```python
from build123d import *

# Parameters (mm, degrees)
BOSS_EXTRUDE1_DEPTH   = 1
SKETCH4_R             = 2
BOSS_EXTRUDE3_DEPTH   = 0.5
SKETCH2_R             = 1
BOSS_EXTRUDE2_DEPTH   = 0.5
CHAMFER1_SIZE         = 0.254
SKETCH5_W             = 0.790640215
SKETCH5_H             = 0.2205187
BOSS_EXTRUDE4_DEPTH   = 1.644
BOSS_EXTRUDE4_2_DEPTH = 1.644
SKETCH7_W             = 0.790640215
SKETCH7_H             = 0.233563057
BOSS_EXTRUDE5_DEPTH   = 0.6
BOSS_EXTRUDE5_2_DEPTH = 0.6
LOFT1_START           = 1.157491545
LOFT1_DEPTH           = 0.790640215
LOFT2_START           = -2.978578696
LOFT2_DEPTH           = 0.790640215
FILLET1_R             = 0.508


# Read off the part's stored shape, not the designer's step: Loft1, Loft2, Mirror1
with BuildPart() as part:
    # Sketch1 → Boss-Extrude1 (new body)
    with BuildSketch(Plane(origin=(0, 0, 0), x_dir=(1, 0, 0), z_dir=(0, 1, 0))):
        Polygon((-3.115223468, 1.972186251), (-2.070005732, 3.017403987), (1.039558796, 3.017403987), (2.084776532, 1.972186251), (2.084776532, -1.137378277), (1.039558796, -2.182596013), (-2.070005732, -2.182596013), (-3.115223468, -1.137378277), align=None)
    extrude(amount=BOSS_EXTRUDE1_DEPTH)

    # Sketch4 → Boss-Extrude3 (add)
    with BuildSketch(Plane(origin=(0, 1, 0), x_dir=(1, 0, 0), z_dir=(0, 1, 0))):
        with Locations(Location((-0.515223468, 0.417403987, 0), (0, 0, 270))):
            Circle(SKETCH4_R)
    extrude(amount=BOSS_EXTRUDE3_DEPTH)

    # Sketch2 → Boss-Extrude2 (add)
    with BuildSketch(Plane(origin=(0, 1.5, 0), x_dir=(1, 0, 0), z_dir=(0, 1, 0))):
        with Locations(Location((-0.515223468, 0.417403987, 0), (0, 0, 270))):
            Circle(SKETCH2_R)
    extrude(amount=BOSS_EXTRUDE2_DEPTH)

    # Chamfer1
    chamfer1_edges = [part.edges().sort_by_distance(p)[0] for p in [
        (-0.515223468, 1.5, -2.417403987),
    ]]
    chamfer(chamfer1_edges, length=CHAMFER1_SIZE)



with BuildPart() as body_2:
    # Sketch5 → Boss-Extrude4 (new body)
    with BuildSketch(Plane.XY.offset(2.182596013)):
        with Locations((-2.583258589, 0.233563057)):
            Rectangle(SKETCH5_W, SKETCH5_H)
    extrude(amount=-BOSS_EXTRUDE4_DEPTH)



with BuildPart() as body_3:
    # Sketch5 → Boss-Extrude4 2 (new body)
    with BuildSketch(Plane.XY.offset(2.182596013)):
        with Locations((1.552811652, 0.233563057)):
            Rectangle(SKETCH5_W, SKETCH5_H)
    extrude(amount=-BOSS_EXTRUDE4_2_DEPTH)


with BuildPart() as body_4:
    # Sketch7 → Boss-Extrude5 (new body)
    with BuildSketch(Plane.XY.offset(2.436596013)):
        with Locations((-2.583258589, 0.116781529)):
            Rectangle(SKETCH7_W, SKETCH7_H)
    extrude(amount=BOSS_EXTRUDE5_DEPTH)


with BuildPart() as body_5:
    # Sketch7 → Boss-Extrude5 2 (new body)
    with BuildSketch(Plane.XY.offset(2.436596013)):
        with Locations((1.552811652, 0.116781529)):
            Rectangle(SKETCH7_W, SKETCH7_H)
    extrude(amount=BOSS_EXTRUDE5_2_DEPTH)


with BuildPart() as part_1:
    add(part.part)

    add(body_3.part)  # Loft1 merges body 3

    add(body_5.part)  # Loft1 merges body 5
    # Loft1 outline → Loft1 (add)
    with BuildSketch(Plane.YZ.offset(LOFT1_START)):
        Polygon((0.233563057, 2.436596013), (0, 2.436596013), (0.123303707, 2.182596013), (0.343822407, 2.182596013), align=None)
    extrude(amount=LOFT1_DEPTH)


with BuildPart() as body_2_1:
    add(body_2.part)

    add(body_4.part)  # Loft2 merges body 4

    add(part_1.part)  # Loft2 merges part
    # Loft2 outline → Loft2 (add)
    with BuildSketch(Plane.YZ.offset(LOFT2_START)):
        Polygon((0.123303707, 2.182596013), (0.343822407, 2.182596013), (0.233563057, 2.436596013), (0, 2.436596013), align=None)
    extrude(amount=LOFT2_DEPTH)

    # Fillet1
    fillet1_edges = [body_2_1.edges().sort_by_distance(p)[0] for p in [
        (1.552811653, 0.343822407, 2.182596013),
        (-2.583258588, 0.343822407, 2.182596013),
        (-2.583258588, 0, 2.436596013),
        (1.552811653, 0, 2.436596013),
        (-2.583258588, 0.233563057, 2.436596013),
        (1.552811653, 0.233563057, 2.436596013),
        (-2.583258588, 0.123303707, 2.182596013),
        (1.552811653, 0.123303707, 2.182596013),
    ]]
    fillet(fillet1_edges, radius=FILLET1_R)

    # Mirror1: body 2 across plane


with BuildPart() as body_2_2:
    add(body_2_1.part)
    add(body_2_1.part.mirror(Plane.XY.offset(-0.417403987)))


solid = body_2_2.part
```
Design review of the part built by this model. Coordinates are the model's own, in mm. A direction names the side the tool comes from. Coordinates: 2 decimals unless noted, no trailing zeros. Write each loop counter-clockwise with the first axis right and the second up, starting at its lowest first coordinate (ties: lowest second). Pieces come first, ordered by that corner, then holes. Notation, with made-up numbers: M 16,64.5 L 30,64.5 A17 ccw 30,97.5 Z; hole C 81,19.25 d6. An arc over 180 degrees is marked long. Answer as a JSON object with one key per item and string values.
Item 1: Insertion check: pin 1 Ø0.6 at (x, z) = (-2.5, -2.5) entering from +Y; pin 2 Ø1.1 at (x, y) = (0, 0.5) entering from +Z. Each pin has a flat end and moves straight along its axis. Give the tip position at first contact, or say it passes through.
Outcome:
{"pin 1": "y = 1", "pin 2": "z = 2.18"}
Item 2: Add section A-A, the plane y = 0.6. Give the boundary of the cut face in (x, z).
Outcome:
{"outline": "M -3.12,-1.97 L -2.07,-3.02 L 1.04,-3.02 L 2.08,-1.97 L 2.08,1.14 L 1.04,2.18 L -2.07,2.18 L -3.12,1.14 Z"}
Item 3: Add section D-D, the plane x = -2.6. Give the boundary of the cut face in (y, z), and give its area (3 significant figures).
Outcome:
{"outline": "M 0,-3.87 L 0.23,-3.87 L 0.23,-3.38 A0.51 cw 0.28,-3.17 L 0.3,-3.11 A0.51 ccw 0.34,-2.91 L 0.34,-2.49 L 1,-2.49 L 1,1.65 L 0.34,1.65 L 0.34,2.08 A0.51 ccw 0.3,2.28 L 0.28,2.34 A0.51 cw 0.23,2.54 L 0.23,3.04 L 0,3.04 L 0,2.55 A0.51 ccw 0.05,2.33 L 0.07,2.29 A0.51 cw 0.12,2.07 L 0.12,1.65 L 0,1.65 L 0,-2.49 L 0.12,-2.49 L 0.12,-2.9 A0.51 cw 0.07,-3.12 L 0.05,-3.17 A0.51 ccw 0,-3.39 Z", "area": "4.77 mm²"}
Item 4: Add section C-C, the plane x = 1.8. Give the boundary of the cut face in (y, z), and give its area (3 significant figures).
Outcome:
{"outline": "M 0,-3.87 L 0.23,-3.87 L 0.23,-3.38 A0.51 cw 0.28,-3.17 L 0.3,-3.11 A0.51 ccw 0.34,-2.91 L 0.34,-2.26 L 1,-2.26 L 1,1.42 L 0.34,1.42 L 0.34,2.08 A0.51 ccw 0.3,2.28 L 0.28,2.34 A0.51 cw 0.23,2.54 L 0.23,3.04 L 0,3.04 L 0,2.55 A0.51 ccw 0.05,2.33 L 0.07,2.29 A0.51 cw 0.12,2.07 L 0.12,1.42 L 0,1.42 L 0,-2.26 L 0.12,-2.26 L 0.12,-2.9 A0.51 cw 0.07,-3.12 L 0.05,-3.17 A0.51 ccw 0,-3.39 Z", "area": "4.41 mm²"}
Item 5: Wall thickness on probe 1 along Y at (x, z) = (0, 1.75); probe 2 along Y at (x, z) = (0.45, -1.5); probe 3 along Z at (x, y) = (0.2, 0.6): over which ranges is each line inside the solid? List them lowest first.
Outcome:
{"probe 1": "0 to 1", "probe 2": "0 to 1.5", "probe 3": "-3.02 to 2.18"}
Item 6: Add section B-B, the plane z = 1.75. Give the boundary of the cut face in (x, y), and give its area (3 significant figures).
Outcome:
{"outline": "M -2.98,0.12 L -2.5,0.12 L -2.5,0 L 1.47,0 L 1.47,0.12 L 1.95,0.12 L 1.95,0.34 L 1.47,0.34 L 1.47,1 L -2.5,1 L -2.5,0.34 L -2.98,0.34 Z", "area": "4.18 mm²"}
Item 7: Machinability: for faces 1 (the flat face through (1, 1, -2)), 2 (the flat face through (2.085, 0.5, -0.4)), 3 (the flat face through (-0.5, 0.5, 2.183)), which of the approach directions +Z, -Z, +X, -X, +Y, -Y give a long, thin tool a straight path to every point of the face, cutting with its end or side? Answer none if there is none.
Outcome:
{"face 1": "+Y", "face 2": "+Z, -Z, +X, +Y, -Y", "face 3": "+Z, +Y, -Y"}
Item 8: Draft analysis for pull direction X (two halves, no side actions). For faces 4 (the flat face through (-0.5, 0.5, -3.017)), 5 (the flat face through (0, 0, 0)), 6 (the cylindrical face through (-0.215, 1.746, 0.536)), state which applies: pulls with the +X half, pulls with the -X half, needs draft (parallel to the pull), parting line crosses it, or undercut.
Outcome:
{"face 4": "undercut", "face 5": "needs draft", "face 6": "parting line crosses it"}
